from build123d import *

# Parameters (mm, degrees)
BOSS_EXTRUDE1_DEPTH = 40.5
SKETCH2_W           = 7.5
SKETCH2_H           = 16
CUT_EXTRUDE1_DEPTH  = 12.5


with BuildPart() as part:
    # Sketch1 → Boss-Extrude1 (new body)
    with BuildSketch(Plane.XY):
        with BuildLine():
            Line((-4, -45.5), (4, -45.5))
            ThreePointArc((4, -45.5), (6.828427125, -44.328427125), (8, -41.5))
            Line((8, -41.5), (8, 41.5))
            ThreePointArc((8, 41.5), (6.828427125, 44.328427125), (4, 45.5))
            Line((4, 45.5), (-4, 45.5))
            ThreePointArc((-4, 45.5), (-6.828427125, 44.328427125), (-8, 41.5))
            Line((-8, 41.5), (-8, -41.5))
            ThreePointArc((-8, -41.5), (-6.828427125, -44.328427125), (-4, -45.5))
        make_face()
    extrude(amount=BOSS_EXTRUDE1_DEPTH)

    # Sketch2 → Cut-Extrude1 (cut)
    with BuildSketch(Plane.XY.offset(40.5)):
        with Locations((0, 7.5)):
            Rectangle(SKETCH2_W, SKETCH2_H)
        with Locations((0, 32.5)):
            Rectangle(SKETCH2_W, SKETCH2_H)
        with Locations((0, -17.5)):
            Rectangle(SKETCH2_W, SKETCH2_H)
    extrude(amount=-CUT_EXTRUDE1_DEPTH, mode=Mode.SUBTRACT)


solid = part.part
Can you work these out from the model? Positions are in its coordinate system, mm. A direction names the side the tool comes from. Give positions to 0.01 mm unless a question says otherwise; leave off trailing zeros. Loops run counter-clockwise (first coordinate to the right, second up) from the corner with the lowest first, then second, coordinate; pieces in that order, holes last. Notation, with made-up numbers: (-15, 17.25) - (33, 17.25) arc R17 ccw to (33, 35.25) - close; hole circle Ø11 at (-33.75, 41.25). An arc over 180 degrees is marked (long way). Return JSON: item names as keys, results as strings.
1. If I drill on line 1 (Y direction, x = 3.25, z = 31); line 2 (Z direction, x = -1, y = 9); line 3 (Y direction, x = -4.25, z = 34.5), over which ranges is the centre line in solid material (lowest first)?
Output values:
{"line 1": "y = -45.5 to -25.5, -9.5 to -0.5, 15.5 to 24.5, 40.5 to 45.5", "line 2": "z = 0 to 28", "line 3": "y = -45.49 to 45.49"}
2. For faces 1 (the face through (3.75, 7, 34)), 2 (the face through (6.797, -44.359, 19.966)), which set-ups out of +Z, -Z, +X, -X, +Y, -Y let a thin tool reach every point of the face, with its end or its side?
Output values:
{"face 1": "+Z", "face 2": "+Z, -Z, +X, -Y"}
3. I want a section at D-D on x = 6.5. Please give me the cut outline in (y, z), and give its area (3 significant figures).
Output values:
{"outline": "(-44.62, 0) - (44.62, 0) - (44.62, 40.5) - (-44.62, 40.5) - close", "area": "3,610 mm²"}
4. I want a section at C-C on x = 0. Please give me the cut outline in (y, z).
Output values:
{"outline": "(-45.5, 0) - (45.5, 0) - (45.5, 40.5) - (40.5, 40.5) - (40.5, 28) - (24.5, 28) - (24.5, 40.5) - (15.5, 40.5) - (15.5, 28) - (-0.5, 28) - (-0.5, 40.5) - (-9.5, 40.5) - (-9.5, 28) - (-25.5, 28) - (-25.5, 40.5) - (-45.5, 40.5) - close"}
5. I want a section at A-A on z = 34.5. Please give me the cut outline in (x, y), and give its area (3 significant figures).
Output values:
{"outline": "(-8, -41.5) arc R4 ccw to (-4, -45.5) - (4, -45.5) arc R4 ccw to (8, -41.5) - (8, 41.5) arc R4 ccw to (4, 45.5) - (-4, 45.5) arc R4 ccw to (-8, 41.5) - close; hole (-3.75, -25.5) - (3.75, -25.5) - (3.75, -9.5) - (-3.75, -9.5) - close; hole (-3.75, -0.5) - (3.75, -0.5) - (3.75, 15.5) - (-3.75, 15.5) - close; hole (-3.75, 24.5) - (3.75, 24.5) - (3.75, 40.5) - (-3.75, 40.5) - close", "area": "1,080 mm²"}
6. I want a section at B-B on y = 13. Please give me the cut outline in (x, z), and give its area (3 significant figures).
Output values:
{"outline": "(-8, 0) - (8, 0) - (8, 40.5) - (3.75, 40.5) - (3.75, 28) - (-3.75, 28) - (-3.75, 40.5) - (-8, 40.5) - close", "area": "554 mm²"}
7. We'd pull the mould along X, two halves only. Please class faces 3 (the face through (-5, 1, 40.5)), 4 (the face through (6.859, 44.297, 19.966)), 5 (the face through (0, -9.5, 34)): +X half, -X half, draft (parallel to the pull), parting line (faces both ways), or undercut.
Output values:
{"face 3": "draft", "face 4": "+X half", "face 5": "undercut"}
8. I'm going to push flat-ended pins straight in: pin 1 Ø6 at (x, y) = (-2, -24) entering from +Z; pin 2 Ø4 at (x, y) = (-0.5, -19.5) entering from +Z. Where does each tip first touch, or does it pass through?
Output values:
{"pin 1": "stops at z = 40.5", "pin 2": "stops at z = 28"}
